Source: three-view drawing plus pictorial views. Frame: mm from the lowest corner of the part. A direction names the side the tool comes from. Round coordinates to 2 decimals unless told otherwise and drop trailing zeros. Loops run counter-clockwise (first coordinate to the right, second up) from the corner with the lowest first, then second, coordinate; pieces in that order, holes last. Notation, with made-up numbers: (14.5, 66.5) -> (47.5, 66.5) arc R28 cw to (47.5, 93.5) -> close; hole circle Ø11 at (85, -31.75). An arc over 180 degrees is marked (long way). Answer as a JSON object with one key per item and string values. Group by question number.
Item 1: Section query C-C on z = 20. Return loops of the section in (x, y).
Item 2: Draft query along Y for the marked faces 4, 5 and 6. Return one class per face: released by +Y, released by -Y, zero draft, split by the parting line, or undercut.
Item 3: Set-up query: the marked faces 1, 2 and 3. Return all of +Z, -Z, +X, -X, +Y, -Y with unobstructed straight access to the full face (end or side cutting, diameter ignored); none if empty.
Item 4: Section query B-B on x = 34. Return loops of the section in (y, z).
Item 5: Pin query (flat end, axial travel): pin 1 (1.7 mm diameter, centred on x = 18.5, z = 15, fed in from -Y); pin 2 (4.5 mm diameter, centred on x = 34, y = 38.5, fed in from +Z); pin 3 (4.5 mm diameter, centred on x = 17, z = 11.5, fed in from +Y); pin 4 (7.5 mm diameter, centred on y = 27.13, z = 20, fed in from -X). Return the tip coordinate at first contact, or that it passes through.
Item 6: Material intervals for line 1 (Y direction, x = 34, z = 2.35); line 2 (Y direction, x = 18.7, z = 20); line 3 (Z direction, x = 29.5, y = 48.5), sorted ascending. Write a range as [from, to].
Item 7: Section query A-A on y = 15.5. Return loops of the section in (x, z).
Item 8: Section query D-D on x = 17.5. Return loops of the section in (y, z).
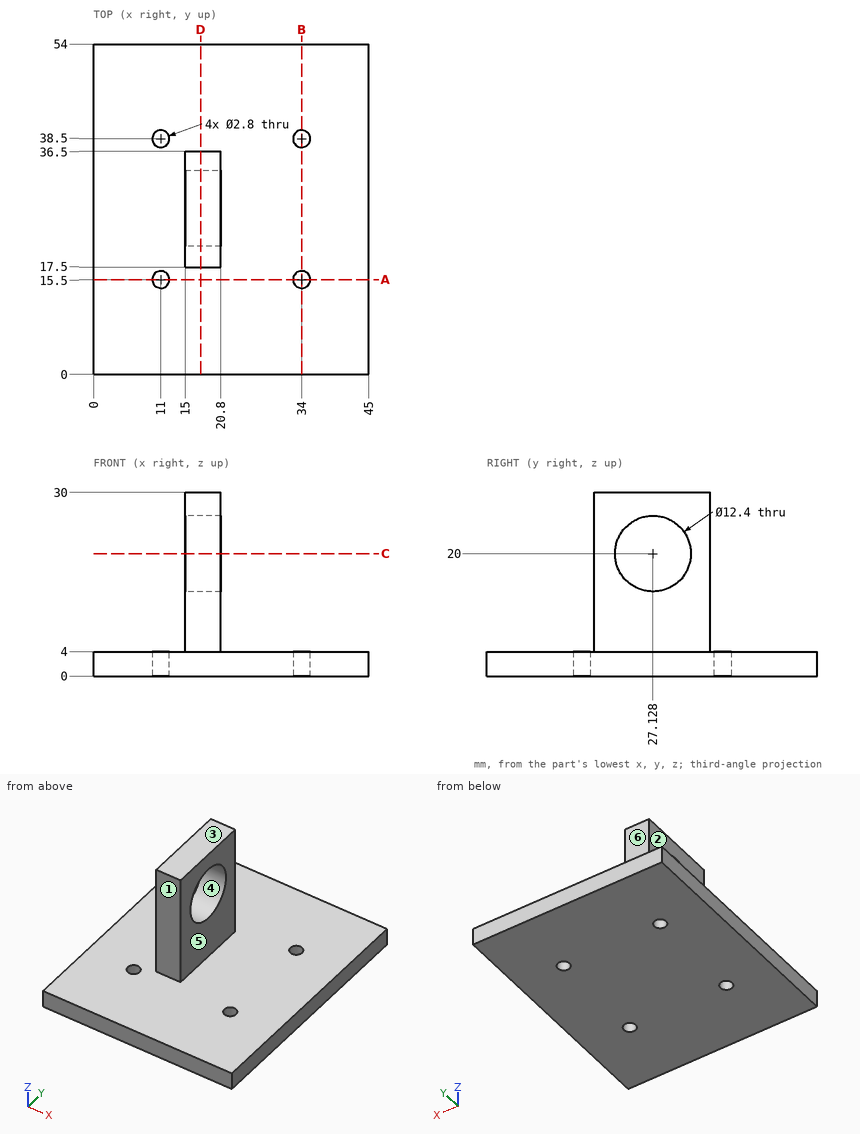
Solved:
{
 "1": {"outline": "(15, 17.5) -> (20.8, 17.5) -> (20.8, 20.93) -> (15, 20.93) -> close; (15, 33.33) -> (20.8, 33.33) -> (20.8, 36.5) -> (15, 36.5) -> close"},
 "2": {"face 4": "undercut", "face 5": "zero draft", "face 6": "released by +Y"},
 "3": {"face 1": "+Z, +X, -X, -Y", "face 2": "+Z, -X, +Y, -Y", "face 3": "+Z, +X, -X, +Y, -Y"},
 "4": {"outline": "(0, 0) -> (14.1, 0) -> (14.1, 4) -> (0, 4) -> close; (16.9, 0) -> (37.1, 0) -> (37.1, 4) -> (16.9, 4) -> close; (39.9, 0) -> (54, 0) -> (54, 4) -> (39.9, 4) -> close"},
 "5": {"pin 1": "y = 17.5", "pin 2": "z = 4", "pin 3": "y = 36.5", "pin 4": "through"},
 "6": {"line 1": "[0, 14.1], [16.9, 37.1], [39.9, 54]", "line 2": "[17.5, 20.93], [33.33, 36.5]", "line 3": "[0, 4]"},
 "7": {"outline": "(0, 0) -> (9.6, 0) -> (9.6, 4) -> (0, 4) -> close; (12.4, 0) -> (32.6, 0) -> (32.6, 4) -> (12.4, 4) -> close; (35.4, 0) -> (45, 0) -> (45, 4) -> (35.4, 4) -> close"},
 "8": {"outline": "(0, 0) -> (54, 0) -> (54, 4) -> (36.5, 4) -> (36.5, 30) -> (17.5, 30) -> (17.5, 4) -> (0, 4) -> close; hole circle Ø12.4 at (27.13, 20)"}
}
